Here's how the part is built. I have some questions about the finished solid (model axes, mm). Face numbers are marked on the shaded views. A direction names the side the tool comes from. Round coordinates to 2 decimals unless told otherwise and drop trailing zeros. Write each loop counter-clockwise with the first axis right and the second up, starting at its lowest first coordinate (ties: lowest second). Pieces come first, ordered by that corner, then holes. Notation, with made-up numbers: (-29.75, 59) - (22.25, 59) arc R25 ccw to (22.25, 94) - close; hole circle Ø11 at (71, 76). An arc over 180 degrees is marked (long way). Use one line per item in the form item = value. Start each with the question number.
1. If I drill on line 1 along Y through (x, z) = (8, 6); line 2 along Z through (x, y) = (10, 5); line 3 along X through (y, z) = (-17, 86), over which ranges is the centre line in solid material (lowest first)?
2. We'd pull the mould along Y, two halves only. Please class the marked faces 3, 4 and 5: +Y half, -Y half, draft (parallel to the pull), parting line (faces both ways), or undercut.
3. Which directions (+Z, -Z, +X, -X, +Y, -Y) give clear straight access to the entire face, cutting with the end or side of a thin tool? Please do the marked faces 1 and 2.
4. I want a section at B-B, the plane z = 158. List the corners of the cut face in (x, y) for me (1 decimal).
5. I want a section at C-C, the plane x = -25.5. List the corners of the cut face in (y, z) for me.
6. Will these pins go through, and if not, where does the flat tip stop? pin 1 (2.5 mm diameter, centred on x = -8.5, y = 43, fed in from +Z); pin 2 (4 mm diameter, centred on x = 35.5, y = 10.5, fed in from +Z); pin 3 (7 mm diameter, centred on x = 22, y = -34.5, fed in from +Z).
7. I want a section at D-D, the plane y = -10. List the corners of the cut face in (x, z) for me.
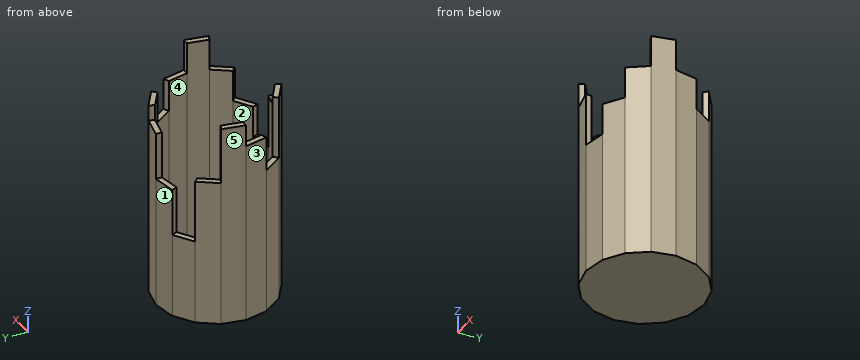
```python
from build123d import *

# Parameters (mm, degrees)
F1_DEPTH  = 152.4
F3_DEPTH  = 25.4
F5_DEPTH  = 50.8
F7_DEPTH  = 12.7
F9_DEPTH  = 63.5
F11_DEPTH = 38.1
F13_DEPTH = 10.16
F15_DEPTH = 5.08
F17_DEPTH = 38.1
F18_DEPTH = 25.4
F20_DEPTH = 7.62
F22_DEPTH = 50.8
F24_DEPTH = 25.4
F26_DEPTH = 25.4
F27_DEPTH = 12.7
F28_DEPTH = 7.62


with BuildPart() as f1:
    # F0 (on Top) → F1 (new body)
    with BuildSketch(Plane.XY):
        Polygon((-0.1432745452, 42.8622605407), (0, 42.8340103128), (0, 47.625), (-18.2252984664, 43.9997627359), (-16.4027686197, 39.5997864623), align=None)
        Polygon((16.3795251941, -39.5436718688), (0, -42.8625), (0, -47.625), (18.2252984664, -43.9997627359), align=None)
        Polygon((-39.5997864623, -16.4027686197), (-42.8625, 0), (-47.625, 0), (-43.9997627359, -18.2252984664), align=None)
        Polygon((39.6860263374, 16.1929990982), (42.8625, 0), (47.625, 0), (43.9997627359, 18.2252984664), (39.5581280192, 16.3855131276), align=None)
        Polygon((39.5997864623, -16.4027686197), (30.3083644086, -30.3083644086), (33.675960454, -33.675960454), (43.9997627359, -18.2252984664), align=None)
        Polygon((-39.5997864623, 16.4027686197), (-30.3083644086, 30.3083644086), (-33.675960454, 33.675960454), (-43.9997627359, 18.2252984664), align=None)
        Polygon((-16.4027686197, -39.5997864623), (-30.3083644086, -30.3083644086), (-33.675960454, -33.675960454), (-18.2252984664, -43.9997627359), align=None)
        Polygon((16.4027686197, 39.5997864623), (30.3083644086, 30.3083644086), (33.675960454, 33.675960454), (18.2252984664, 43.9997627359), align=None)
        Polygon((0, -47.625), (0, -42.8625), (-16.4027686197, -39.5997864623), (-18.2252984664, -43.9997627359), align=None)
        Polygon((0, 47.625), (0, 42.8340103128), (16.4027686197, 39.5997864623), (18.2252984664, 43.9997627359), align=None)
        Polygon((-33.675960454, -33.675960454), (-30.3083644086, -30.3083644086), (-39.5997864623, -16.4027686197), (-43.9997627359, -18.2252984664), align=None)
        Polygon((33.675960454, 33.675960454), (30.3083644086, 30.3083644086), (39.5581280192, 16.3855131276), (43.9997627359, 18.2252984664), align=None)
        Polygon((33.675960454, -33.675960454), (30.3083644086, -30.3083644086), (16.684655354, -39.481846233), (16.3795251941, -39.5436718688), (18.2252984664, -43.9997627359), align=None)
        Polygon((-33.675960454, 33.675960454), (-30.3083644086, 30.3083644086), (-16.4027686197, 39.5997864623), (-18.2252984664, 43.9997627359), align=None)
        Polygon((-47.625, 0), (-42.8625, 0), (-39.5997864623, 16.4027686197), (-43.9997627359, 18.2252984664), align=None)
        Polygon((47.625, 0), (42.8625, 0), (39.5997864623, -16.4027686197), (43.9997627359, -18.2252984664), align=None)
    extrude(amount=F1_DEPTH)

    # F2 (on face) → F3 (cut)
    with BuildSketch(Plane.XY.offset(152.4)):
        Polygon((39.6860263374, 16.1929990982), (43.9997627359, 18.2252984664), (33.675960454, 33.675960454), (30.3083644086, 30.3083644086), align=None)
    extrude(amount=-F3_DEPTH, mode=Mode.SUBTRACT)

    # F4 (on face) → F5 (cut)
    with BuildSketch(Plane.XY.offset(152.4)):
        Polygon((-0.1432745452, 42.8622605407), (0, 47.625), (-18.2252984664, 43.9997627359), (-16.4027686197, 39.5997864623), align=None)
    extrude(amount=-F5_DEPTH, mode=Mode.SUBTRACT)

    # F6 (on face) → F7 (cut)
    with BuildSketch(Plane.XY.offset(152.4)):
        Polygon((16.4027686197, 39.5997864623), (18.2252984664, 43.9997627359), (0, 47.625), (-0.1432745452, 42.8622605407), align=None)
    extrude(amount=-F7_DEPTH, mode=Mode.SUBTRACT)

    # F8 (on face) → F9 (cut)
    with BuildSketch(Plane.XY.offset(152.4)):
        Polygon((-18.2252984664, 43.9997627359), (-33.675960454, 33.675960454), (-30.3083644086, 30.3083644086), (-16.4027686197, 39.5997864623), align=None)
    extrude(amount=-F9_DEPTH, mode=Mode.SUBTRACT)

    # F10 (on face) → F11 (cut)
    with BuildSketch(Plane.XY.offset(152.4)):
        Polygon((-33.675960454, 33.675960454), (-43.9997627359, 18.2252984664), (-39.5997864623, 16.4027686197), (-30.3083644086, 30.3083644086), align=None)
    extrude(amount=-F11_DEPTH, mode=Mode.SUBTRACT)

    # F12 (on face) → F13 (cut)
    with BuildSketch(Plane.XY.offset(152.4)):
        Polygon((-42.8625, 0), (-47.625, 0), (-43.9997627359, -18.2252984664), (-39.5997864623, -16.4027686197), align=None)
    extrude(amount=-F13_DEPTH, mode=Mode.SUBTRACT)

    # F14 (on face) → F15 (join)
    with BuildSketch(Plane(origin=(0, 0, 0), x_dir=(1, 0, 0), z_dir=(0, 0, -1))):
        Polygon((-18.2252984664, -43.9997627359), (0, -47.625), (18.2252984664, -43.9997627359), (33.675960454, -33.675960454), (43.9997627359, -18.2252984664), (47.625, 0), (43.9997627359, 18.2252984664), (33.675960454, 33.675960454), (18.2252984664, 43.9997627359), (0, 47.625), (-18.2252984664, 43.9997627359), (-33.675960454, 33.675960454), (-43.9997627359, 18.2252984664), (-47.625, 0), (-43.9997627359, -18.2252984664), (-33.675960454, -33.675960454), align=None)
        Polygon((30.3083644086, -30.3083644086), (16.4027686197, -39.5997864623), (-0.1432745452, -42.8622605407), (-16.4027686197, -39.5997864623), (-30.3083644086, -30.3083644086), (-39.5997864623, -16.4027686197), (-42.8625, 0), (-39.5997864623, 16.4027686197), (-30.3083644086, 30.3083644086), (-16.4027686197, 39.5997864623), (0, 42.8625), (16.684655354, 39.481846233), (30.3083644086, 30.3083644086), (39.5997864623, 16.4027686197), (42.8625, 0), (39.6860263374, -16.1929990982), align=None, mode=Mode.SUBTRACT)
        Polygon((-0.1432745452, -42.8622605407), (16.4027686197, -39.5997864623), (30.3083644086, -30.3083644086), (39.6860263374, -16.1929990982), (42.8625, 0), (39.5997864623, 16.4027686197), (30.3083644086, 30.3083644086), (16.684655354, 39.481846233), (0, 42.8625), (-16.4027686197, 39.5997864623), (-30.3083644086, 30.3083644086), (-39.5997864623, 16.4027686197), (-42.8625, 0), (-39.5997864623, -16.4027686197), (-30.3083644086, -30.3083644086), (-16.4027686197, -39.5997864623), align=None)
    extrude(amount=F15_DEPTH)

    # F16 (on face) → F17 (cut)
    with BuildSketch(Plane.XY.offset(152.4)):
        Polygon((-33.675960454, -33.675960454), (-30.3083644086, -30.3083644086), (-39.5997864623, -16.4027686197), (-43.9997627359, -18.2252984664), align=None)
    extrude(amount=-F17_DEPTH, mode=Mode.SUBTRACT)

    # F18 (cut): a face of the model
    f18_faces = [f1.faces().sort_by_distance(p)[0] for p in [
        (-24.6758616972, 36.9300368148, 88.9),
    ]]
    extrude(f18_faces, amount=-F18_DEPTH, mode=Mode.SUBTRACT)

    # F19 (on face) → F20 (cut)
    with BuildSketch(Plane.XY.offset(152.4)):
        Polygon((-16.4027686197, -39.5997864623), (-18.2252984664, -43.9997627359), (0, -47.625), (0, -42.8625), align=None)
    extrude(amount=-F20_DEPTH, mode=Mode.SUBTRACT)

    # F21 (on face) → F22 (cut)
    with BuildSketch(Plane.XY.offset(152.4)):
        Polygon((0, -47.625), (18.2252984664, -43.9997627359), (16.684655354, -39.481846233), (0, -42.8625), align=None)
    extrude(amount=-F22_DEPTH, mode=Mode.SUBTRACT)

    # F23 (on face) → F24 (cut)
    with BuildSketch(Plane.XY.offset(152.4)):
        Polygon((18.2252984664, -43.9997627359), (33.675960454, -33.675960454), (30.3083644086, -30.3083644086), (16.684655354, -39.481846233), align=None)
    extrude(amount=-F24_DEPTH, mode=Mode.SUBTRACT)

    # F25 (on face) → F26 (join)
    with BuildSketch(Plane.XY.offset(152.4)):
        Polygon((43.9997627359, -18.2252984664), (47.625, 0), (42.8625, 0), (39.5997864623, -16.4027686197), align=None)
    extrude(amount=F26_DEPTH)

    # F27 (add): a face of the model
    f27_faces = [f1.faces().sort_by_distance(p)[0] for p in [
        (-24.6758616972, -36.9300368148, 152.4),
    ]]
    extrude(f27_faces, amount=F27_DEPTH)

    # F28 (add): a face of the model
    f28_faces = [f1.faces().sort_by_distance(p)[0] for p in [
        (-43.561948599, 8.6650103235, 152.4),
    ]]
    extrude(f28_faces, amount=F28_DEPTH)


solid = f1.part
```
Model answer:
q1.line_1 = -46.03 to -41.24, 41.26 to 46.03
q1.line_2 = -5.08 to 0
q1.line_3 = -44.24 to -39.2, 39.2 to 44.24
q2.face_3 = -Y half
q2.face_4 = undercut
q2.face_5 = +Y half
q3.face_1 = +Z, -Z, -X, +Y
q3.face_2 = +Z
q4.outline = (-47.6, 0) - (-42.9, 0) - (-39.6, 16.4) - (-44, 18.2) - close; (-33.7, -33.7) - (-18.2, -44) - (-16.4, -39.6) - (-30.3, -30.3) - close; (39.6, -16.4) - (44, -18.2) - (47.6, 0) - (42.9, 0) - close
q5.outline = (-39.14, -5.08) - (39.14, -5.08) - (39.14, 63.5) - (33.52, 63.5) - (33.52, 0) - (-33.52, 0) - (-33.52, 165.1) - (-39.14, 165.1) - close
q6.pin_1 = 101.6
q6.pin_2 = 0
q6.pin_3 = 127
q7.outline = (-45.64, -5.08) - (45.64, -5.08) - (45.64, 177.8) - (40.87, 177.8) - (40.87, 0) - (-40.87, 0) - (-40.87, 142.24) - (-45.64, 142.24) - close
